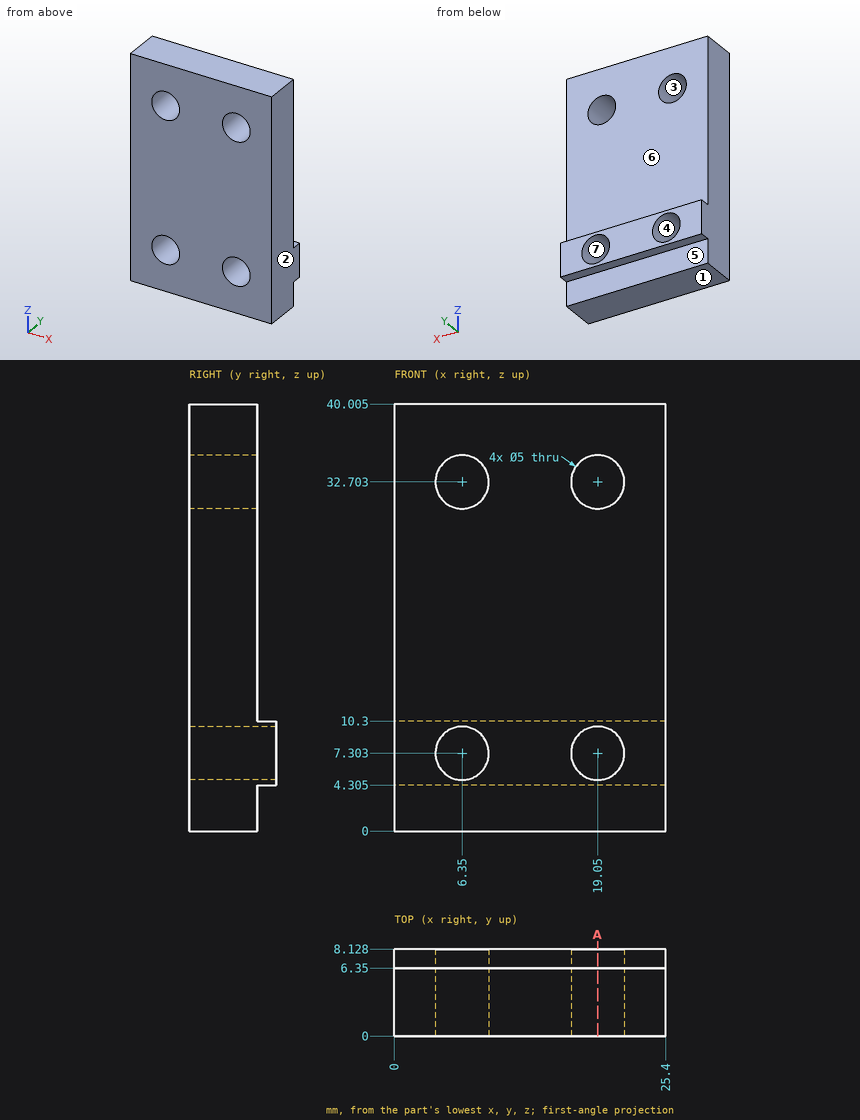
Drawing for the job (mm, zero at the part's lowest x, y, z). A direction names the side the tool comes from. Give positions to 0.01 mm unless a question says otherwise; leave off trailing zeros. Use CSV: the item, a comma, the result in double quotes.
Item 1: Pin check, flat tips, straight feed: P1, Ø4.5, axis at x = 6.35, z = 7.3, coming from the +Y side; P2, Ø6, axis at x = 6.35, z = 32.7, coming from the +Y side; P3, Ø3, axis at y = 2, z = 14.5, coming from the -X side; P4, Ø0.9, axis at x = 11, y = 7.5, coming from the -Z side (1 decimal). Stop position of each tip, or through.
Taken from the geometry:
P1,"passes through"
P2,"stops at y = 6.35"
P3,"stops at x = 0"
P4,"stops at z = 4.3"
Item 2: Pull direction Z, two halves, no side cores. Call the marked faces 1, 2, 3 and 4: +Z half, -Z half, draft (parallel to the pull), parting line (faces both ways), or undercut.
Taken from the geometry:
face 1,"-Z half"
face 2,"draft"
face 3,"undercut"
face 4,"undercut"
Item 3: Slice it at A-A on x = 19.05. State how many separate pieces and enclosed holes the cut face has, plus the area to 3 significant figures.
Taken from the geometry:
separate pieces,"3"
enclosed holes,"0"
area,"192 mm²"
Item 4: Drill centre lines: probe 1 along Z at (x, y) = (6.35, 5.25) (1 decimal); probe 2 along X at (y, z) = (2, 32.5); probe 3 along X at (y, z) = (4, 9) (1 decimal). Where is each one in solid material? Low to high.
Taken from the geometry:
probe 1,"z = 0 to 4.8, 9.8 to 30.2, 35.2 to 40"
probe 2,"x = 0 to 3.86, 8.84 to 16.56, 21.54 to 25.4"
probe 3,"x = 0 to 4.5, 8.2 to 17.2, 20.9 to 25.4"
Item 5: Which spindle directions (+Z, -Z, +X, -X, +Y, -Y) get a long thin tool onto all of the face, cutting with end or side? Do the marked faces 5, 6 and 7. Say none if no direction does.
Taken from the geometry:
face 5,"-Z, +X, -X, +Y"
face 6,"+Z, +X, -X, +Y"
face 7,"+Y, -Y"
